```python
from build123d import *

# Parameters (mm, degrees)
SKETCH1_W           = 15.85
SKETCH1_H           = 15.85
BOSS_EXTRUDE1_DEPTH = 3.15
SHELL1_T            = -1.5
SKETCH2_R           = 3.225
SKETCH2_R_2         = 2.425
BOSS_EXTRUDE2_DEPTH = 1.45


with BuildPart() as part:
    # Sketch1 → Boss-Extrude1 (new body)
    with BuildSketch(Plane(origin=(0, 0, 0), x_dir=(1, 0, 0), z_dir=(0, 1, 0))):
        Rectangle(SKETCH1_W, SKETCH1_H)
    extrude(amount=-BOSS_EXTRUDE1_DEPTH)

    # Shell1
    shell1_openings = [part.faces().sort_by_distance(p)[0] for p in [
        (0, -3.15, 0),
    ]]
    offset(amount=SHELL1_T, openings=shell1_openings, kind=Kind.INTERSECTION)

    # Sketch2 → Boss-Extrude2 (add)
    with BuildSketch(Plane.XZ.offset(1.5)):
        with Locations(Location((0, 0, 0), (0, 0, 90))):
            Circle(SKETCH2_R)
        with Locations(Location((0, 0, 0), (0, 0, 90))):
            Circle(SKETCH2_R_2, mode=Mode.SUBTRACT)
    extrude(amount=BOSS_EXTRUDE2_DEPTH)


solid = part.part
```
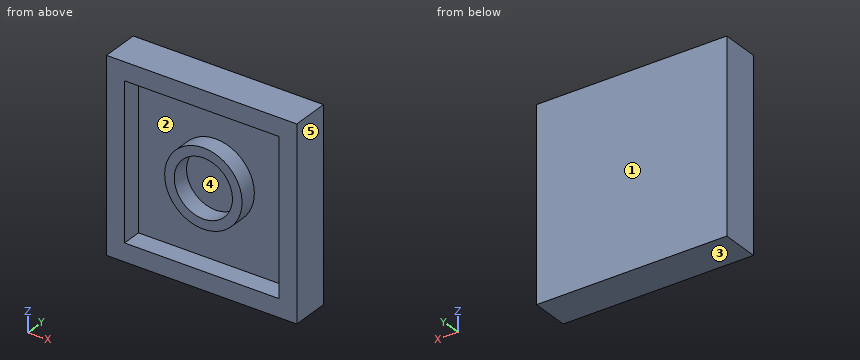
Work out the finished part from the listing and answer in its coordinate system (mm). Face numbers are marked on the shaded views. A direction names the side the tool comes from. Give positions to 0.01 mm unless a question says otherwise; leave off trailing zeros. Order: outer loops, then holes, each group sorted by start corner. A loop starts at its lowest first (then second) coordinate and runs counter-clockwise, first axis right, second up. Notation, with made-up numbers: (29.5, 10) - (67.5, 10) arc R15 cw to (67.5, 16) - close; hole circle Ø1 at (73, 45). An arc over 180 degrees is marked (long way). One line per item, written item: value. Start each with the question number.
1. Section A-A, the plane y = -2 is taken. Write down the section's boundary in (x, z) (3 decimals).
2. Section B-B, the plane z = 0 is taken. Write down the section's boundary in (x, y) (3 decimals), then the cut area to 3 significant figures.
3. Section C-C, the plane x = 4.25 is taken. Write down the section's boundary in (y, z) (3 decimals).
4. Which of the six approach directions +Z, -Z, +X, -X, +Y, -Y give full straight-line access (tool end or side, diameter ignored) to the marked faces 1 and 2?
5. Consider line 1 (X direction, y = -2.05, z = 0) (3 decimals); line 2 (Z direction, x = 5.25, y = -2.75) (3 decimals). Determine where each line is inside the solid, lowest interval first.
6. For a pull along Z with two mould halves and no side action, classify the marked faces 3, 4 and 5 as released by +Z, released by -Z, zero draft, split by the parting line, or undercut.
7. Each of these flat-tipped pins is pushed along its axis until it touches: pin 1 Ø5 at (x, z) = (-1, 1) entering from -Y; pin 2 Ø1.5 at (x, z) = (0.5, -1) entering from -Y. Where does it stop, or does it pass through?
8. Section D-D, the plane z = -6 is taken. Write down the section's boundary in (x, y) (3 decimals).
Filled sheet:
1. outline: (-7.925, -7.925) - (7.925, -7.925) - (7.925, 7.925) - (-7.925, 7.925) - close; circle Ø6.45 at (0, 0); hole (-6.425, -6.425) - (6.425, -6.425) - (6.425, 6.425) - (-6.425, 6.425) - close; hole circle Ø4.85 at (0, 0)
2. outline: (-7.925, -3.15) - (-6.425, -3.15) - (-6.425, -1.5) - (-3.225, -1.5) - (-3.225, -2.95) - (-2.425, -2.95) - (-2.425, -1.5) - (2.425, -1.5) - (2.425, -2.95) - (3.225, -2.95) - (3.225, -1.5) - (6.425, -1.5) - (6.425, -3.15) - (7.925, -3.15) - (7.925, 0) - (-7.925, 0) - close
2. area: 31.0 mm²
3. outline: (-3.15, -7.925) - (0, -7.925) - (0, 7.925) - (-3.15, 7.925) - (-3.15, 6.425) - (-1.5, 6.425) - (-1.5, -6.425) - (-3.15, -6.425) - close
4. face 1: +Z, -Z, +X, -X, +Y
4. face 2: -Y
5. line 1: -7.925 to -6.425, -3.225 to -2.425, 2.425 to 3.225, 6.425 to 7.925
5. line 2: -7.925 to -6.425, 6.425 to 7.925
6. face 3: released by -Z
6. face 4: undercut
6. face 5: zero draft
7. pin 1: y = -2.95
7. pin 2: y = -1.5
8. outline: (-7.925, -3.15) - (-6.425, -3.15) - (-6.425, -1.5) - (6.425, -1.5) - (6.425, -3.15) - (7.925, -3.15) - (7.925, 0) - (-7.925, 0) - close
